Can you work these out from the drawing? Everything is in mm from the part's minimum corner. A direction names the side the tool comes from. Round coordinates to 2 decimals unless told otherwise and drop trailing zeros. Order: outer loops, then holes, each group sorted by start corner. A loop starts at its lowest first (then second) coordinate and runs counter-clockwise, first axis right, second up. Notation, with made-up numbers: (21.25, -15) - (42.25, -15) arc R15 ccw to (42.25, 14) - close; hole circle Ø3 at (26.25, -18.75). An arc over 180 degrees is marked (long way). Write item = value, one per line.
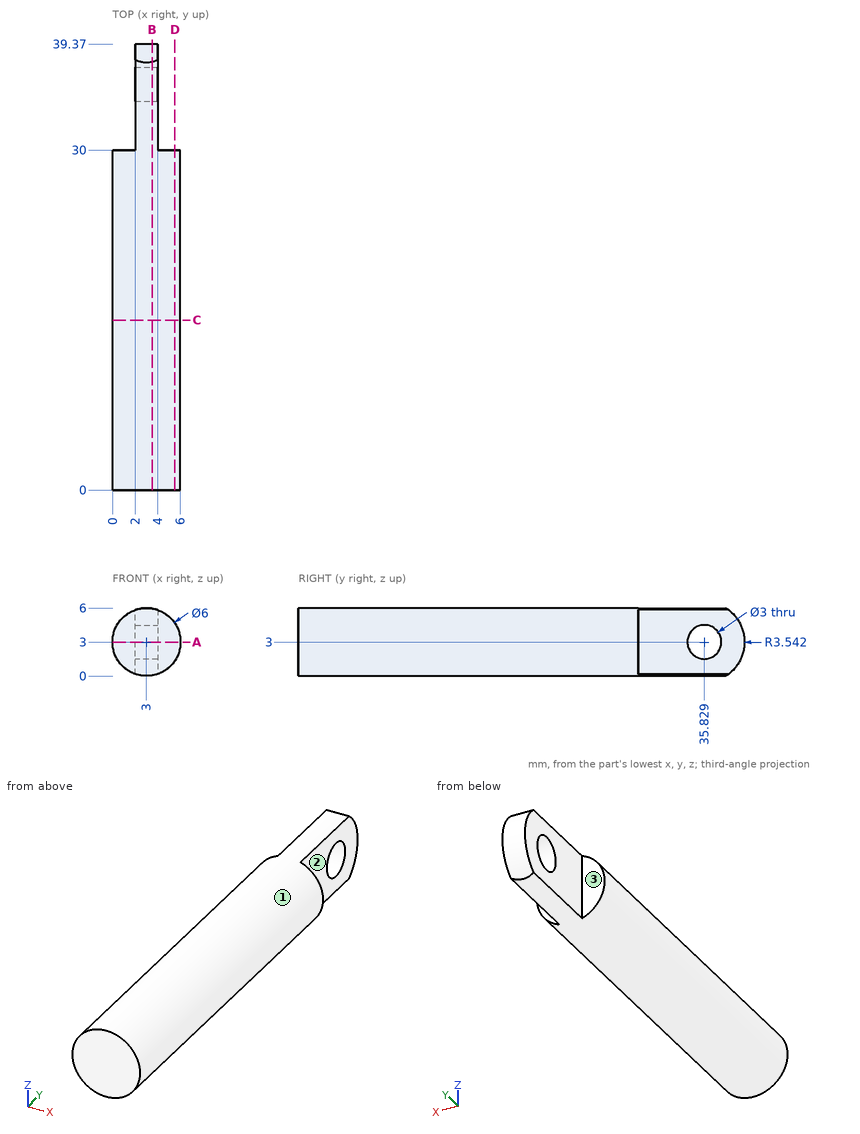
(1) Will these pins go through, and if not, where does the flat tip stop? P1, Ø3, axis at y = 35.5, z = 3, coming from the -X side; P2, Ø1.6, axis at x = 1, z = 4.5, coming from the +Y side; P3, Ø2, axis at x = 1, y = 8.5, coming from the +Z side.
Computed:
P1 = 2
P2 = 30
P3 = 5.83
(2) If I drill on line 1 (Z direction, x = 4, y = 14.5); line 2 (X direction, y = 37.5, z = 5.5); line 3 (Y direction, x = 5.75, z = 2), over which ranges is the centre line in solid material (lowest first)? Write a range as from..to.
Computed:
line_1 = 0.17..5.83
line_2 = 2..4
line_3 = 0..30
(3) If we section it at B-B (x = 3.5): Write out the boundary of the cut face in (y, z), plus the area to 3 significant figures.
Computed:
outline = (0, 0.04) - (37.78, 0.04) arc R3.54 ccw to (37.78, 5.96) - (0, 5.96) - close; hole circle Ø3 at (35.83, 3)
area = 223 mm^2
(4) On a 3-axis mill with a long thin cutter (end or side, diameter ignored), from which of +Z, -Z, +X, -X, +Y, -Y can I reach the whole of each face in a straight line? I mean the marked faces 1, 2 and 3. Say none if no direction works.
Computed:
face_1 = +Y, -Y
face_2 = +Z, -Z, +X, +Y
face_3 = +Z, -Z, -X, +Y
(5) If we section it at D-D (x = 5.5): Write out the boundary of the cut face in (y, z).
Computed:
outline = (0, 1.34) - (30, 1.34) - (30, 4.66) - (0, 4.66) - close
(6) If we section it at C-C (y = 15): Write out the boundary of the cut face in (x, z), plus the area to 3 significant figures.
Computed:
outline = circle Ø6 at (3, 3)
area = 28.3 mm^2
(7) If we section it at A-A (z = 3): Write out the boundary of the cut face in (x, y), plus the area to 3 significant figures.
Computed:
outline = (0, 0) - (6, 0) - (6, 30) - (4, 30) - (4, 34.33) - (2, 34.33) - (2, 30) - (0, 30) - close; (2, 37.33) - (4, 37.33) - (4, 39.37) - (2, 39.37) - close
area = 193 mm^2
